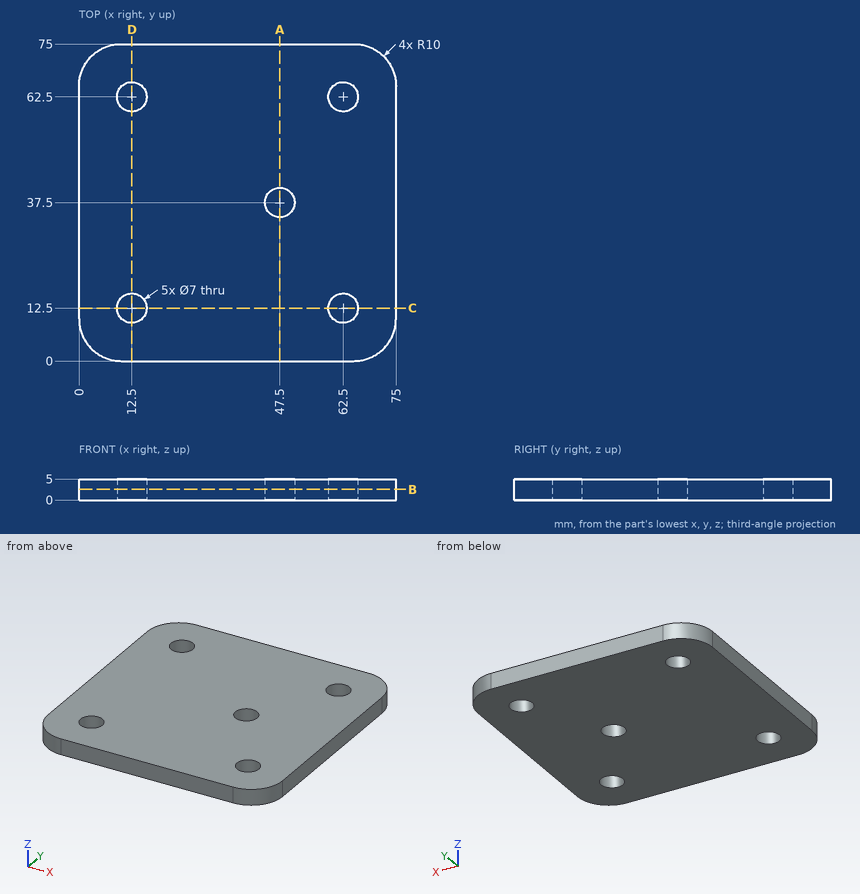
Job drawing, mm, ordinate dimensions from the low corner. One solid piece. Round coordinates to 2 decimals unless told otherwise and drop trailing zeros. Write each loop counter-clockwise with the first axis right and the second up, starting at its lowest first coordinate (ties: lowest second). Pieces come first, ordered by that corner, then holes. Notation, with made-up numbers: M 26.5,-4.5 L 47.5,-4.5 A11 cw 47.5,11.5 Z; hole C 35.25,-39 d6. An arc over 180 degrees is marked long. Return JSON: item names as keys, results as strings. Group by question number.
(1) Saw through at C-C on y = 12.5. Write the cut outline in (x, z).
(2) Saw through at A-A on x = 47.5. Write the cut outline in (y, z).
(3) Pin check, flat tip, straight feed: pin 1 Ø3 at (x, z) = (23, 2) entering from -Y. Stop position of the tip, or through.
(4) Saw through at B-B on z = 2.55. Write the cut outline in (x, y).
(5) Drill centre lines: probe 1 along Y at (x, z) = (62.5, 2.25); probe 2 along Y at (x, z) = (47.5, 3.95); probe 3 along X at (y, z) = (40.5, 2.5). Where is each one in solid material? Low to high.
Returned:
{
 "1": {"outline": "M 0,0 L 9,0 L 9,5 L 0,5 Z; M 16,0 L 59,0 L 59,5 L 16,5 Z; M 66,0 L 75,0 L 75,5 L 66,5 Z"},
 "2": {"outline": "M 0,0 L 34,0 L 34,5 L 0,5 Z; M 41,0 L 75,0 L 75,5 L 41,5 Z"},
 "3": {"pin 1": "y = 0"},
 "4": {"outline": "M 0,10 A10 ccw 10,0 L 65,0 A10 ccw 75,10 L 75,65 A10 ccw 65,75 L 10,75 A10 ccw 0,65 Z; hole C 12.5,12.5 d7; hole C 12.5,62.5 d7; hole C 47.5,37.5 d7; hole C 62.5,12.5 d7; hole C 62.5,62.5 d7"},
 "5": {"probe 1": "0 to 9, 16 to 59, 66 to 75", "probe 2": "0 to 34, 41 to 75", "probe 3": "0 to 45.7, 49.3 to 75"}
}
